The model under review builds one solid part; all positions refer to its coordinate system, in mm. Face numbers are marked on the shaded views. Round coordinates to 2 decimals unless told otherwise and drop trailing zeros. Order: outer loops, then holes, each group sorted by start corner. A loop starts at its lowest first (then second) coordinate and runs counter-clockwise, first axis right, second up.
```python
from build123d import *

# Parameters (mm, degrees)
SKIZZE1_R                       = 2
AUFSATZ_LINEAR_AUSTRAGEN1_DEPTH = 15
VERRUNDUNG1_R                   = 5
SKIZZE2_R                       = 2
SCHNITT_LINEAR_AUSTRAGEN1_DEPTH = 29.442925307


with BuildPart() as part:
    # Skizze1 → Aufsatz-Linear austragen1 (new body)
    with BuildSketch(Plane(origin=(0, 0, 0), x_dir=(1, 0, 0), z_dir=(0, 1, 0))):
        with BuildLine():
            Line((0, 12), (0, -12))
            Line((0, -12), (10, -12))
            Line((10, -12), (10, 2))
            ThreePointArc((10, 2), (17.071067812, 19.071067812), (0, 12))
        make_face()
        with Locations(Location((10, 12, 0), (0, 0, 270))):
            Circle(SKIZZE1_R, mode=Mode.SUBTRACT)
    extrude(amount=AUFSATZ_LINEAR_AUSTRAGEN1_DEPTH)

    # Verrundung1
    verrundung1_edges = [part.edges().sort_by_distance(p)[0] for p in [
        (5, 15, 12),
        (5, 0, 12),
    ]]
    fillet(verrundung1_edges, radius=VERRUNDUNG1_R)

    # Skizze2 → Schnitt-Linear austragen1 (cut, through all)
    with BuildSketch(Plane(origin=(10, 0, 0), x_dir=(0, 0, -1), z_dir=(1, 0, 0))):
        with Locations((-6, 7.5)):
            Circle(SKIZZE2_R)
    extrude(amount=-SCHNITT_LINEAR_AUSTRAGEN1_DEPTH, mode=Mode.SUBTRACT)


solid = part.part
```
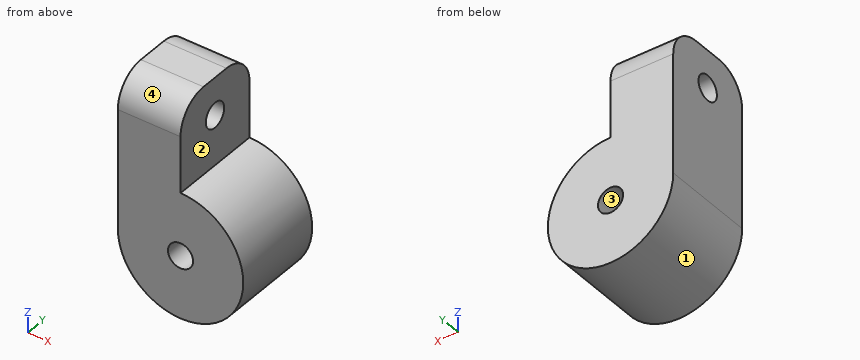
(1) Consider section B-B (x = 8.75). Write out the cut boundary in (y, z), and give its area (3 significant figures).
Data:
outline: (0, -21.92) - (15, -21.92) - (15, -13.56) - (0, -13.56) - close; (0, -10.44) - (15, -10.44) - (15, 7) arc R5 ccw to (10, 12) - (5, 12) arc R5 ccw to (0, 7) - close; hole circle Ø4 at (7.5, 6)
area: 439 mm2
(2) Consider section C-C (z = 6). Write out the cut boundary in (x, y).
Data:
outline: (0, 0) - (10, 0) - (10, 5.5) - (0, 5.5) - close; (0, 9.5) - (10, 9.5) - (10, 15) - (0, 15) - close
(3) Draft analysis for pull direction X (two halves, no side actions). For the marked faces 1, 2, 3 and 4, state which applies: pulls with the +X half, pulls with the -X half, needs draft (parallel to the pull), parting line crosses it, or undercut.
Data:
face 1: parting line crosses it
face 2: pulls with the +X half
face 3: undercut
face 4: needs draft
(4) Consider section A-A (y = 7.5). Write out the cut boundary in (x, z), and give its area (3 significant figures).
Data:
outline: (0, -12) arc R10 ccw (long way) to (10, -2) - (10, 4) - (0, 4) - close; (0, 8) - (10, 8) - (10, 12) - (0, 12) - close; hole circle Ø4 at (10, -12)
area: 423 mm2
(5) Consider section D-D (x = 11.5). Write out the cut boundary in (y, z), and give its area (3 significant figures).
Data:
outline: (0, -21.89) - (15, -21.89) - (15, -13.32) - (0, -13.32) - close; (0, -10.68) - (15, -10.68) - (15, -2.11) - (0, -2.11) - close
area: 257 mm2
(6) To check wall thickness, follow probe 1 along Y at (x, z) = (2.5, 6); probe 2 along X at (y, z) = (3, 7.5); probe 3 along X at (y, z) = (9.75, -12). State the ranges of each line that lie inside material, in increasing order.
Data:
probe 1: y = 0 to 5.5, 9.5 to 15
probe 2: x = 0 to 10
probe 3: x = 0 to 8, 12 to 20
(7) Insertion check: pin 1 (4 mm diameter, centred on y = 9.5, z = 4.5, fed in from +X); pin 2 (5 mm diameter, centred on y = 13, z = -16, fed in from +X); pin 3 (4 mm diameter, centred on y = 3.5, z = -5.5, fed in from +X). Each pin has a flat end and moves straight along its axis. Give the tip position at first contact, or say it passes through.
Data:
pin 1: stops at x = 10
pin 2: stops at x = 19.89
pin 3: stops at x = 18.93
